Could you check a few things on this drawing? It's one solid part, dimensions in mm from its lowest x, y, z. A direction names the side the tool comes from. Give positions to 0.01 mm unless a question says otherwise; leave off trailing zeros. Loops run counter-clockwise (first coordinate to the right, second up) from the corner with the lowest first, then second, coordinate; pieces in that order, holes last. Notation, with made-up numbers: (52.5, 80.5) - (75.5, 80.5) arc R19 ccw to (75.5, 104.5) - close; hole circle Ø5 at (86, 26.5). An arc over 180 degrees is marked (long way). Write each question's results on one line, items separated by ' | '. Start each with the question number.
(1) Suppose I cut it at B-B (y = 19.5). Please give me the cut outline in (x, z) (1 decimal), and give its area (3 significant figures).
(2) If we mould it in two halves opening along X, with no side actions, what happens to the marked faces 4, 5 and 6? For each: released by +X, released by -X, zero draft, split by the parting line, or undercut.
(3) For pin 1 (5 mm diameter, centred on y = 14.5, z = 9.5, fed in from -X); pin 2 (1 mm diameter, centred on x = 16.5, z = 3.5, fed in from -Y) (1 decimal); pin 3 (4 mm diameter, centred on x = 4, z = 7, fed in from -Y); pin 4 (3 mm diameter, centred on x = 12.7, y = 19.05, fed in from -Z), each with a flat end and sliding along its axis, tell me the tip position at first contact or that it passes through.
(4) I need wall thicknesses on line 1 (Y direction, x = 12.7, z = 9.45) (1 decimal); line 2 (Y direction, x = 11.5, z = 6) (1 decimal); line 3 (Y direction, x = 11.25, z = 8.75) (1 decimal). Which ranges of each line are inside material? Lowest first, please.
(5) On a 3-axis mill with a long thin cutter (end or side, diameter ignored), from which of +Z, -Z, +X, -X, +Y, -Y can I reach the whole of each face in a straight line? I mean the marked faces 1, 2 and 3. Say none if no direction works.
(6) Suppose I cut it at A-A (x = 12.7). Count the separate pieces of the cut face and the enclosed holes in it, and give its area (3 significant figures).
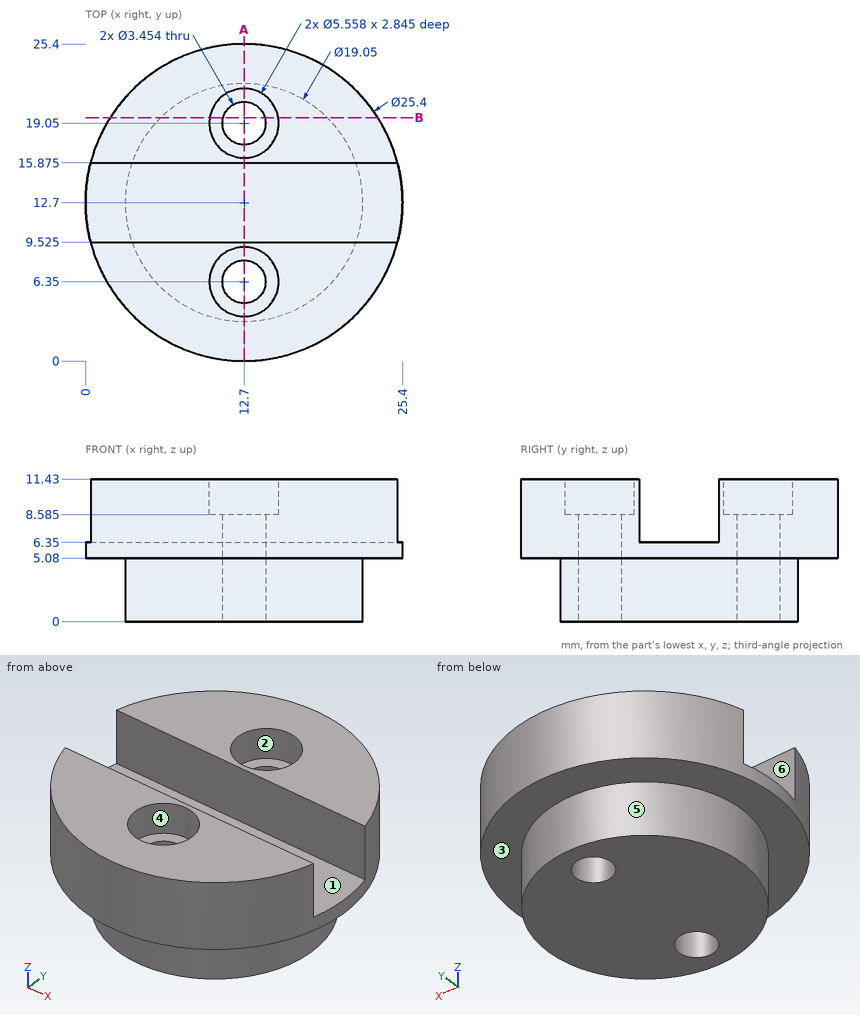
Output values:
1) outline: (2, 5.1) - (6, 5.1) - (6, 0) - (11, 0) - (11, 8.6) - (10, 8.6) - (10, 11.4) - (2, 11.4) - close; (14.4, 0) - (19.4, 0) - (19.4, 5.1) - (23.4, 5.1) - (23.4, 11.4) - (15.4, 11.4) - (15.4, 8.6) - (14.4, 8.6) - close | area: 160 mm2
2) face 4: undercut | face 5: split by the parting line | face 6: zero draft
3) pin 1: x = 0.4 | pin 2: y = 3.8 | pin 3: y = 1.91 | pin 4: through
4) line 1: 0 to 3.6, 9.1 to 9.5, 15.9 to 16.3, 21.8 to 25.4 | line 2: 0.1 to 5.1, 7.6 to 17.8, 20.3 to 25.3 | line 3: 0.1 to 4, 8.7 to 9.5, 15.9 to 16.7, 21.4 to 25.3
5) face 1: +Z, +X, -X | face 2: +Z | face 3: -Z
6) separate pieces: 3 | enclosed holes: 0 | area: 135 mm2
